Verification items for the finished model (mm, model axes). Give positions to 0.01 mm unless a question says otherwise; leave off trailing zeros. Order: outer loops, then holes, each group sorted by start corner. A loop starts at its lowest first (then second) coordinate and runs counter-clockwise, first axis right, second up.
(1) Mould release check, pull along X, two halves, no side actions. Record for faces 1 (the face through (-30, -1, 1)), 2 (the face through (-26.3, -38.4, 1)), 3 (the face through (0, 1, 2)): pulls with the +X half, pulls with the -X half, needs draft (parallel to the pull), parting line crosses it, or undercut.
(2) Sectioned sample at B-B on x = -27.5. Record the cut outline in (y, z), plus the area to 3 significant figures.
(3) Scan line: L1, parallel to Y at x = 27.5, z = 0.55. Record every from-to range of solid material in increasing order.
(4) Sectioned sample at A-A on y = -37.5. Record the cut outline in (x, z).
```python
from build123d import *

# Parameters (mm, degrees)
CROQUIS1_W              = 60
CROQUIS1_H              = 80
SALIENTE_EXTRUIR1_DEPTH = 2
CORTAR_EXTRUIR1_REACH   = 4
CROQUIS2_R              = 1.5


with BuildPart() as part:
    # Croquis1 → Saliente-Extruir1 (new body)
    with BuildSketch(Plane.XY):
        Rectangle(CROQUIS1_W, CROQUIS1_H)
    extrude(amount=SALIENTE_EXTRUIR1_DEPTH)

    # Croquis2 → Cortar-Extruir1 (cut, up to next)
    with BuildSketch(Plane(origin=(0, 0, 0), x_dir=(-1, 0, 0), z_dir=(0, 0, -1)), mode=Mode.PRIVATE) as cortar_extruir1_sk1:
        with Locations((27.5, -37.5)):
            Circle(CROQUIS2_R)
    cortar_extruir1_tool1 = extrude(cortar_extruir1_sk1.sketch, amount=-CORTAR_EXTRUIR1_REACH, mode=Mode.PRIVATE) & part.part
    add(cortar_extruir1_tool1.solids().sort_by_distance((-27.5, -37.5, 0))[0], mode=Mode.SUBTRACT)
    # Croquis2 → Cortar-Extruir1 (cut, up to next)
    with BuildSketch(Plane(origin=(0, 0, 0), x_dir=(-1, 0, 0), z_dir=(0, 0, -1)), mode=Mode.PRIVATE) as cortar_extruir1_sk2:
        with Locations((-27.5, -37.5)):
            Circle(CROQUIS2_R)
    cortar_extruir1_tool2 = extrude(cortar_extruir1_sk2.sketch, amount=-CORTAR_EXTRUIR1_REACH, mode=Mode.PRIVATE) & part.part
    add(cortar_extruir1_tool2.solids().sort_by_distance((27.5, -37.5, 0))[0], mode=Mode.SUBTRACT)
    # Croquis2 → Cortar-Extruir1 (cut, up to next)
    with BuildSketch(Plane(origin=(0, 0, 0), x_dir=(-1, 0, 0), z_dir=(0, 0, -1)), mode=Mode.PRIVATE) as cortar_extruir1_sk3:
        with Locations((-27.5, 37.5)):
            Circle(CROQUIS2_R)
    cortar_extruir1_tool3 = extrude(cortar_extruir1_sk3.sketch, amount=-CORTAR_EXTRUIR1_REACH, mode=Mode.PRIVATE) & part.part
    add(cortar_extruir1_tool3.solids().sort_by_distance((27.5, 37.5, 0))[0], mode=Mode.SUBTRACT)
    # Croquis2 → Cortar-Extruir1 (cut, up to next)
    with BuildSketch(Plane(origin=(0, 0, 0), x_dir=(-1, 0, 0), z_dir=(0, 0, -1)), mode=Mode.PRIVATE) as cortar_extruir1_sk4:
        with Locations((27.5, 37.5)):
            Circle(CROQUIS2_R)
    cortar_extruir1_tool4 = extrude(cortar_extruir1_sk4.sketch, amount=-CORTAR_EXTRUIR1_REACH, mode=Mode.PRIVATE) & part.part
    add(cortar_extruir1_tool4.solids().sort_by_distance((-27.5, 37.5, 0))[0], mode=Mode.SUBTRACT)


solid = part.part
```
Ans:
1. face 1: pulls with the -X half
1. face 2: undercut
1. face 3: needs draft
2. outline: (-40, 0) - (-39, 0) - (-39, 2) - (-40, 2) - close; (-36, 0) - (36, 0) - (36, 2) - (-36, 2) - close; (39, 0) - (40, 0) - (40, 2) - (39, 2) - close
2. area: 148 mm2
3. L1: y = -40 to -39, -36 to 36, 39 to 40
4. outline: (-30, 0) - (-29, 0) - (-29, 2) - (-30, 2) - close; (-26, 0) - (26, 0) - (26, 2) - (-26, 2) - close; (29, 0) - (30, 0) - (30, 2) - (29, 2) - close
